The listing builds one solid part. Answer for the finished solid, in the listing's coordinates (mm). A direction names the side the tool comes from. Coordinates: 2 decimals unless noted, no trailing zeros. Write each loop counter-clockwise with the first axis right and the second up, starting at its lowest first coordinate (ties: lowest second). Pieces come first, ordered by that corner, then holes. Notation, with made-up numbers: M -26.5,-29.5 L -21.5,-29.5 A8 cw -21.5,-22.5 Z; hole C 16,85.5 d4. An arc over 180 degrees is marked long. Put each result on its own line as item: value. Start each with the question number.
```python
from build123d import *

# Parameters (mm, degrees)
SKETCH1_R           = 15
BOSS_EXTRUDE1_DEPTH = 5
CUT_EXTRUDE1_DEPTH  = 2.75
CIRPATTERN1_COUNT   = 4
SKETCH2_R           = 4
CUT_EXTRUDE2_DEPTH  = 22.794494718
SKETCH2_3_R         = 6
SKETCH2_3_R_2       = 4
CUT_EXTRUDE3_DEPTH  = 3.5


with BuildPart() as part:
    # Sketch1 → Boss-Extrude1 (new body)
    with BuildSketch(Plane.XY):
        Circle(SKETCH1_R)
    extrude(amount=BOSS_EXTRUDE1_DEPTH)

    # Sketch1_3 → Cut-Extrude1 (cut)
    with BuildSketch(Plane.XY):
        with BuildLine():
            Line((-5.625, 11.864469015), (-5.625, 10.075))
            ThreePointArc((-5.625, 10.075), (-5.441941738, 9.633058262), (-5, 9.45))
            Line((-5, 9.45), (5, 9.45))
            ThreePointArc((5, 9.45), (5.441941738, 9.633058262), (5.625, 10.075))
            Line((5.625, 10.075), (5.625, 11.864469015))
            ThreePointArc((5.625, 11.864469015), (5.520732191, 12.210103193), (5.242718447, 12.440414112))
            ThreePointArc((5.242718447, 12.440414112), (4.087012875, 12.866480706), (2.897283889, 13.185436893))
            ThreePointArc((2.897283889, 13.185436893), (2.83061126, 13.196348557), (2.763150376, 13.2))
            Line((2.763150376, 13.2), (-2.763150376, 13.2))
            ThreePointArc((-2.763150376, 13.2), (-2.83061126, 13.196348557), (-2.897283889, 13.185436893))
            ThreePointArc((-2.897283889, 13.185436893), (-4.087012875, 12.866480706), (-5.242718447, 12.440414112))
            ThreePointArc((-5.242718447, 12.440414112), (-5.520732191, 12.210103193), (-5.625, 11.864469015))
        make_face()
    cut_extrude1 = extrude(amount=CUT_EXTRUDE1_DEPTH, mode=Mode.SUBTRACT)

    # CirPattern1: Cut-Extrude1 ×4 about axis
    cirpattern1_axis = Axis((0, 0, 0), (0, 0, 1))
    for i in range(1, CIRPATTERN1_COUNT):
        add(cut_extrude1.rotate(cirpattern1_axis, i * 360 / CIRPATTERN1_COUNT), mode=Mode.SUBTRACT)

    # Sketch2 → Cut-Extrude2 (cut, through all)
    with BuildSketch(Plane(origin=(0, 0, 0), x_dir=(-1, 0, 0), z_dir=(0, 0, -1))):
        Circle(SKETCH2_R)
    extrude(amount=-CUT_EXTRUDE2_DEPTH, mode=Mode.SUBTRACT)

    # Sketch2_3 → Cut-Extrude3 (cut)
    with BuildSketch(Plane(origin=(0, 0, 0), x_dir=(-1, 0, 0), z_dir=(0, 0, -1))):
        Circle(SKETCH2_3_R)
        Circle(SKETCH2_3_R_2, mode=Mode.SUBTRACT)
    extrude(amount=-CUT_EXTRUDE3_DEPTH, mode=Mode.SUBTRACT)


solid = part.part
```
1) A cutting plane is placed at C-C on z = 1. State how many separate pieces and enclosed holes the cut face has, then the cut area to 3 significant figures.
2) A cutting plane is placed at A-A on y = 0. Write down the section's boundary in (x, z), then the cut area to 3 significant figures.
3) For faces 3 (the face through (0, 7, 0)), 4 (the face through (6, 0, 2)), determine the directions among +Z, -Z, +X, -X, +Y, -Y from which every point of the face is accessible in a straight line to the end or side of a thin tool.
4) Determine the mould class of faces 1 (the face through (3, -3, 5)), 2 (the face through (0, -13.2, 1)) for opening direction X: +X half, -X half, draft (parallel to the pull), parting line (faces both ways), or undercut.
5) A cutting plane is placed at D-D on z = 4.4. Write down the section's boundary in (x, y).
6) Given pin 1 Ø3.5 at (x, y) = (0, -1.5) entering from -Z; pin 2 Ø0.8 at (y, z) = (-1.5, 1) entering from -X; pin 3 Ø2 at (x, z) = (11, 2) entering from -Y; pin 4 Ø1.4 at (y, z) = (-11, 1) entering from +X, each flat-ended and moving along its own axis, determine where each tip first touches the part or whether it passes through.
7) Straight lines are drawn through the part: probe 1 along Y at (x, z) = (0, 1.2); probe 2 along Y at (x, z) = (0, 4.25); probe 3 along X at (y, z) = (4.75, 0.7). For each, find the intervals that lie inside material, in ascending order.
Answers follow:
1. separate pieces: 1
1. enclosed holes: 5
1. area: 435 mm²
2. outline: M -15,0 L -13.2,0 L -13.2,2.75 L -9.45,2.75 L -9.45,0 L -6,0 L -6,3.5 L -4,3.5 L -4,5 L -15,5 Z; M 4,3.5 L 6,3.5 L 6,0 L 9.45,0 L 9.45,2.75 L 13.2,2.75 L 13.2,0 L 15,0 L 15,5 L 4,5 Z
2. area: 75.4 mm²
3. face 3: -Z, +X, -X, +Y, -Y
3. face 4: -Z
4. face 1: draft
4. face 2: undercut
5. outline: C 0,0 d30; hole C 0,0 d8
6. pin 1: passes through
6. pin 2: stops at x = -14.96
6. pin 3: stops at y = -11.18
6. pin 4: stops at x = 10.9
7. probe 1: y = -15 to -13.2, -9.45 to -6, 6 to 9.45, 13.2 to 15
7. probe 2: y = -15 to -4, 4 to 15
7. probe 3: x = -14.23 to -12.64, -9.45 to -3.67, 3.67 to 9.45, 12.64 to 14.23
